For this review, take the finished solid that the model builds, in its own axes (mm). Coordinates: 2 decimals unless noted, no trailing zeros. Loops run counter-clockwise (first coordinate to the right, second up) from the corner with the lowest first, then second, coordinate; pieces in that order, holes last. Notation, with made-up numbers: (67, -31.5) - (102, -31.5) arc R11 ccw to (102, -23.5) - close; hole circle Ø2 at (-24.5, -13.5). An arc over 180 degrees is marked (long way). Use one line per item in the form item = value. Start each with the question number.
1. For pin 1 Ø0.6 at (y, z) = (24, 4.5) entering from -X; pin 2 Ø1 at (x, z) = (-79, 6) entering from +Y; pin 3 Ø2 at (y, z) = (10.5, 4) entering from -X, all flat-tipped, find the tip position at first contact; note any pin that passes through.
2. Add section B-B on x = -100. Give the boundary of the cut face in (y, z), and give its area (3 significant figures).
3. To check wall thickness, follow probe 1 along Y at (x, z) = (-322, 2.5); probe 2 along X at (y, z) = (-23, 7.25); probe 3 along X at (y, z) = (-29, 2). State the ranges of each line that lie inside material, in increasing order.
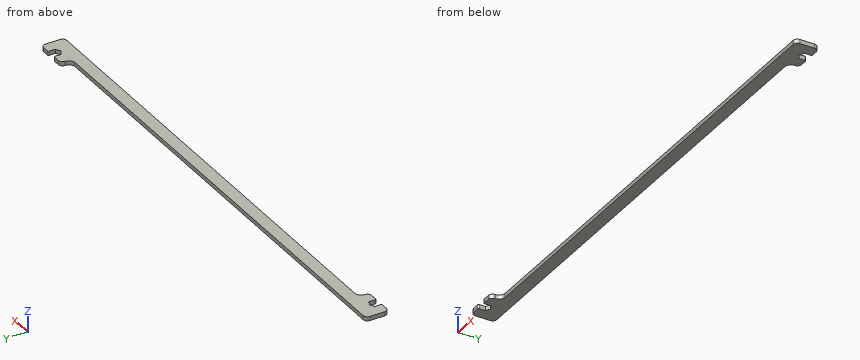
```python
from build123d import *

# Parameters (mm, degrees)
PAD_DEPTH = 8


with BuildPart() as part:
    # Sketch → Pad (new body)
    with BuildSketch(Plane.XY):
        with BuildLine():
            Line((-428.25, 12), (428.25, 12))
            ThreePointArc((428.25, 12), (436.735281, 15.514719), (440.25, 24))
            Line((440.25, 24), (440.25, 24.5))
            ThreePointArc((448.25, 32.5), (442.593146, 30.156854), (440.25, 24.5))
            Line((448.25, 32.5), (460.45, 32.5))
            ThreePointArc((462.45, 30.5), (461.864214, 31.914214), (460.45, 32.5))
            Line((462.45, 29.369358), (462.45, 30.5))
            Line((462.45, 29.369358), (462.45, 18.630642))
            Line((462.45, 18.630642), (471.75, 13.261285))
            Line((471.75, 13.261285), (481.05, 18.630642))
            Line((481.05, 18.630642), (481.05, 29.369358))
            Line((481.05, 29.369358), (481.05, 30.5))
            ThreePointArc((483.05, 32.5), (481.635786, 31.914214), (481.05, 30.5))
            Line((483.05, 32.5), (495.25, 32.5))
            ThreePointArc((503.25, 24.5), (500.906854, 30.156854), (495.25, 32.5))
            Line((503.25, 24.5), (503.25, -4))
            ThreePointArc((495.25, -12), (500.906854, -9.656854), (503.25, -4))
            Line((428.25, -12), (495.25, -12))
            Line((-428.25, -12), (428.25, -12))
            ThreePointArc((-428.25, -12), (-436.735281, -15.514719), (-440.25, -24))
            Line((-440.25, -24), (-440.25, -24.5))
            ThreePointArc((-448.25, -32.5), (-442.593146, -30.156854), (-440.25, -24.5))
            Line((-460.95, -32.5), (-448.25, -32.5))
            ThreePointArc((-462.95, -30.5), (-462.364214, -31.914214), (-460.95, -32.5))
            Line((-462.95, -29.080682), (-462.95, -30.5))
            Line((-462.95, -29.080682), (-462.95, -18.919318))
            Line((-462.95, -18.919318), (-471.75, -13.838635))
            Line((-471.75, -13.838635), (-480.55, -18.919318))
            Line((-480.55, -18.919318), (-480.55, -29.080682))
            Line((-480.55, -29.080682), (-480.55, -30.5))
            ThreePointArc((-482.55, -32.5), (-481.135786, -31.914214), (-480.55, -30.5))
            Line((-495.25, -32.5), (-482.55, -32.5))
            ThreePointArc((-503.25, -24.5), (-500.906854, -30.156854), (-495.25, -32.5))
            Line((-503.25, 4), (-503.25, -24.5))
            ThreePointArc((-495.25, 12), (-500.906854, 9.656854), (-503.25, 4))
            Line((-428.25, 12), (-495.25, 12))
        make_face()
    extrude(amount=PAD_DEPTH)


solid = part.part
```
Conclusion:
q1.pin_1 = 440.25
q1.pin_2 = 12
q1.pin_3 = -501.06
q2.outline = (-12, 0) - (12, 0) - (12, 8) - (-12, 8) - close
q2.area = 192 mm^2
q3.probe_1 = -12 to 12
q3.probe_2 = -503.25 to -480.55, -462.95 to -440.21
q3.probe_3 = -501.86 to -480.55, -462.95 to -441.64
